```python
from build123d import *

# Parameters (mm, degrees)
SKETCH1_R           = 3
BOSS_EXTRUDE1_DEPTH = 4.85
CHAMFER1_SIZE       = 0.25


with BuildPart() as part:
    # Sketch1 → Boss-Extrude1 (new body)
    with BuildSketch(Plane(origin=(0, 0, 0), x_dir=(0, 0, -1), z_dir=(1, 0, 0))):
        with BuildLine():
            Line((4.729124762, 2.901358129), (0.351828076, 5.537031425))
            ThreePointArc((0.351828076, 5.537031425), (0.103101508, 5.608602318), (-0.148087464, 5.546221245))
            Line((-0.148087464, 5.546221245), (-4.619295838, 3.073207764))
            ThreePointArc((-4.619295838, 3.073207764), (-4.805641333, 2.893589685), (-4.877212226, 2.644863117))
            Line((-4.877212226, 2.644863117), (-4.971123914, -2.463823661))
            ThreePointArc((-4.971123914, -2.463823661), (-4.908742841, -2.715012633), (-4.729124762, -2.901358129))
            Line((-4.729124762, -2.901358129), (-0.351828076, -5.537031425))
            ThreePointArc((-0.351828076, -5.537031425), (-0.103101508, -5.608602318), (0.148087464, -5.546221245))
            Line((0.148087464, -5.546221245), (4.619295838, -3.073207764))
            ThreePointArc((4.619295838, -3.073207764), (4.805641333, -2.893589685), (4.877212226, -2.644863117))
            Line((4.877212226, -2.644863117), (4.971123914, 2.463823661))
            ThreePointArc((4.971123914, 2.463823661), (4.908742841, 2.715012633), (4.729124762, 2.901358129))
        make_face()
        Circle(SKETCH1_R, mode=Mode.SUBTRACT)
    extrude(amount=BOSS_EXTRUDE1_DEPTH)

    # Chamfer1
    chamfer1_edges = [part.edges().sort_by_distance(p)[0] for p in [
        (4.85, 5.608602318, -0.103101508),
        (0, -0.090519728, -4.92416807),
        (0, -2.893589685, -4.805641333),
        (0, -4.309714505, -2.383691651),
        (0, -5.608602318, 0.103101508),
        (0, -4.219194777, 2.540476419),
        (0, -2.715012633, 4.908742841),
        (4.85, 4.309714505, 2.383691651),
        (0, 0.090519728, 4.92416807),
        (0, 2.893589685, 4.805641333),
        (0, 4.309714505, 2.383691651),
        (0, 5.608602318, -0.103101508),
        (0, 4.219194777, -2.540476419),
        (0, 2.715012633, -4.908742841),
        (4.85, 2.893589685, 4.805641333),
        (4.85, 0.090519728, 4.92416807),
        (4.85, -2.715012633, 4.908742841),
        (4.85, -4.219194777, 2.540476419),
        (4.85, -5.608602318, 0.103101508),
        (0, 0, 3),
        (4.85, 0, 3),
        (4.85, -4.309714505, -2.383691651),
        (4.85, -2.893589685, -4.805641333),
        (4.85, -0.090519728, -4.92416807),
        (4.85, 2.715012633, -4.908742841),
        (4.85, 4.219194777, -2.540476419),
    ]]
    chamfer(chamfer1_edges, length=CHAMFER1_SIZE)


solid = part.part
```
Can you work these out from the model? Positions are in its coordinate system, mm. Give positions to 0.01 mm unless a question says otherwise; leave off trailing zeros. Order: outer loops, then holes, each group sorted by start corner. A loop starts at its lowest first (then second) coordinate and runs counter-clockwise, first axis right, second up. Notation, with made-up numbers: M 26.5,-5 L 68.5,-5 A32 ccw 68.5,33 Z; hole C -27.75,72.5 d11. An arc over 180 degrees is marked long. Write item = value, one per line. Start each with the question number.
Q1. We'd pull the mould along Z, two halves only. Please class faces 1 (the cylindrical face through (2, 0, 3)), 2 (the flat face through (4.85, -1.116, 3.214)), 3 (the flat face through (2.4, 4.3, 2.4)), 4 (the flat face through (2.4, -4.3, -2.4)): pulls with the +Z half, pulls with the -Z half, needs draft (parallel to the pull), parting line crosses it, or undercut.
Q2. Suppose I cut it at B-B (x = 1.5). Write out the boundary of the cut face in (y, z), plus the area to 3 significant figures.
Q3. Will these pins go through, and if not, where does the flat tip stop? pin 1 Ø1 at (x, z) = (4, 1) entering from +Y; pin 2 Ø1.5 at (x, y) = (4.5, 0) entering from -Z; pin 3 Ø3 at (y, z) = (-1.5, -0.5) entering from -X.
Q4. I need wall thicknesses on probe 1 along Y at (x, z) = (3.5, -2); probe 2 along Y at (x, z) = (3.05, -1); probe 3 along Z at (x, y) = (3.5, 2.75). Which ranges of each line are inside material? Lowest first, please. Write a range as [from, to].
Q5. Suppose I cut it at A-A (y = 0). Write out the boundary of the cut face in (x, z).
Check result:
q1.face_1 = undercut
q1.face_2 = needs draft
q1.face_3 = pulls with the +Z half
q1.face_4 = pulls with the -Z half
q2.outline = M -5.55,-0.15 L -3.07,-4.62 A0.5 ccw -2.64,-4.88 L 2.46,-4.97 A0.5 ccw 2.9,-4.73 L 5.54,-0.35 A0.5 ccw 5.55,0.15 L 3.07,4.62 A0.5 ccw 2.64,4.88 L -2.46,4.97 A0.5 ccw -2.9,4.73 L -5.54,0.35 A0.5 ccw Z; hole C 0,0 d6
q2.area = 55.7 mm2
q3.pin_1 = 5.35
q3.pin_2 = -4.94
q3.pin_3 = 0.17
q4.probe_1 = [-4.52, -2.24], [2.24, 4.54]
q4.probe_2 = [-5.08, -2.83], [2.83, 5.15]
q4.probe_3 = [-4.89, -1.2], [1.2, 4.86]
q5.outline = M 0,-4.68 L 0.25,-4.93 L 4.6,-4.93 L 4.85,-4.68 L 4.85,-3.25 L 4.6,-3 L 0.25,-3 L 0,-3.25 Z; M 0,3.25 L 0.25,3 L 4.6,3 L 4.85,3.25 L 4.85,4.68 L 4.6,4.93 L 0.25,4.93 L 0,4.68 Z
